```python
from build123d import *

# Parameters (mm, degrees)
SKETCH4_R                = 3
BOSS_EXTRUDE2_DEPTH      = 15
BOSS_EXTRUDE2_DEPTH_BACK = 15
SKETCH5_R                = 3
BOSS_EXTRUDE3_DEPTH      = 15
SKETCH6_R                = 2
CUT_EXTRUDE1_DEPTH       = 31
SKETCH7_R                = 2
CUT_EXTRUDE2_DEPTH       = 15


with BuildPart() as part:
    # Sketch4 → Boss-Extrude2 (new body, two sides)
    with BuildSketch(Plane(origin=(0, 0, 0), x_dir=(1, 0, 0), z_dir=(0, 1, 0))) as boss_extrude2_sk:
        Circle(SKETCH4_R)
    extrude(amount=BOSS_EXTRUDE2_DEPTH)
    extrude(boss_extrude2_sk.sketch, amount=-BOSS_EXTRUDE2_DEPTH_BACK)

    # Sketch5 → Boss-Extrude3 (add)
    with BuildSketch(Plane(origin=(0, 0, 0), x_dir=(0, 0, -1), z_dir=(1, 0, 0))):
        Circle(SKETCH5_R)
    extrude(amount=BOSS_EXTRUDE3_DEPTH)

    # Sketch6 → Cut-Extrude1 (cut, through all)
    with BuildSketch(Plane.XZ.offset(15)):
        Circle(SKETCH6_R)
    extrude(amount=-CUT_EXTRUDE1_DEPTH, mode=Mode.SUBTRACT)

    # Sketch7 → Cut-Extrude2 (cut)
    with BuildSketch(Plane(origin=(15, 0, 0), x_dir=(0, 0, -1), z_dir=(1, 0, 0))):
        Circle(SKETCH7_R)
    extrude(amount=-CUT_EXTRUDE2_DEPTH, mode=Mode.SUBTRACT)


solid = part.part
```
The model under review builds one solid part; all positions refer to its coordinate system, in mm. A direction names the side the tool comes from. Round coordinates to 2 decimals unless told otherwise and drop trailing zeros. Write each loop counter-clockwise with the first axis right and the second up, starting at its lowest first coordinate (ties: lowest second). Pieces come first, ordered by that corner, then holes.
(1) Mouldability with a two-part tool opening along Z and no side actions: class faces 1 (the cylindrical face through (7.605, -0.766, -1.847)), 2 (the flat face through (1, 15, 2)), 3 (the cylindrical face through (-3, 0, 0)) as +Z half, -Z half, draft (parallel to the pull), parting line (faces both ways), or undercut.
(2) Insertion check: pin 1 (3 mm diameter, centred on x = 3.5, y = -5.5, fed in from +Z); pin 2 (3 mm diameter, centred on y = -9.5, z = 1, fed in from +X); pin 3 (1.5 mm diameter, centred on y = 6, z = -1.5, fed in from +X); pin 4 (8 mm diameter, centred on x = 4.5, y = 2.5, fed in from -Z). Each pin has a flat end and moves straight along its axis. Give the tip position at first contact, or say it passes through.
(3) Machinability: for faces 4 (the cylindrical face through (-2, 0, 0)), 5 (the cylindrical face through (9, 0, 3)), which of the approach directions +Z, -Z, +X, -X, +Y, -Y give a long, thin tool a straight path to every point of the face, cutting with its end or side? Answer none if there is none.
(4) We need section D-D on x = 6.5. Give the boundary of the cut face in (y, z).
(5) We need section A-A on z = 0. Give the boundary of the cut face in (x, y), and give its area (3 significant figures).
(6) We need section C-C on x = -1.5. Give the boundary of the cut face in (y, z).
(7) Wall thickness on L1, parallel to Y at x = 7, z = 0; L2, parallel to X at y = 8.5, z = -1.75: over which ranges is each line inside the solid? List them lowest first.
(8) We need section B-B on y = 0. Give the boundary of the cut face in (x, z), and give its area (3 significant figures).
Findings below:
1. face 1: undercut
1. face 2: draft
1. face 3: parting line
2. pin 1: stops at z = 2.24
2. pin 2: stops at x = 3
2. pin 3: stops at x = 2.9
2. pin 4: stops at z = -3
3. face 4: +Y, -Y
3. face 5: +X
4. outline: circle Ø6 at (0, 0); hole circle Ø4 at (0, 0)
5. outline: (-3, -15) - (-2, -15) - (-2, 15) - (-3, 15) - close; (2, -15) - (3, -15) - (3, -3) - (15, -3) - (15, -2) - (2, -2) - close; (2, 2) - (15, 2) - (15, 3) - (3, 3) - (3, 15) - (2, 15) - close
5. area: 80.0 mm2
6. outline: (-15, -2.6) - (15, -2.6) - (15, -1.32) - (-15, -1.32) - close; (-15, 1.32) - (15, 1.32) - (15, 2.6) - (-15, 2.6) - close
7. L1: y = -3 to -2, 2 to 3
7. L2: x = -2.44 to -0.97, 0.97 to 2.44
8. outline: (0, -3) - (15, -3) - (15, -2) - (0, -2) arc R2 cw to (0, 2) - (15, 2) - (15, 3) - (0, 3) arc R3 ccw to start
8. area: 37.9 mm2
